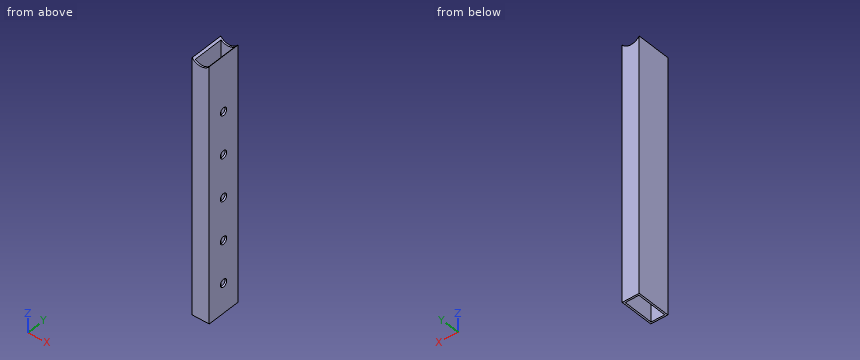
```python
from build123d import *

# Parameters (mm, degrees)
SKETCH_1_W          = 20
SKETCH_1_H          = 40
SKETCH_1_W_2        = 16
SKETCH_1_H_2        = 36
EXTRUDE_1_DEPTH     = 300
SKETCH_2_R          = 12.5
CUT_EXTRUDE_1_DEPTH = 40
SKETCH_3_R          = 4.5
CUT_EXTRUDE_2_DEPTH = 2


with BuildPart() as part:
    # Эскиз1 → Бобышка-Вытянуть1 (new body)
    with BuildSketch(Plane.XY):
        Rectangle(SKETCH_1_W, SKETCH_1_H)
        Rectangle(SKETCH_1_W_2, SKETCH_1_H_2, mode=Mode.SUBTRACT)
    extrude(amount=EXTRUDE_1_DEPTH)

    # Эскиз2 → Вырез-Вытянуть1 (cut)
    with BuildSketch(Plane(origin=(0, 20, 0), x_dir=(1, 0, 0), z_dir=(0, 1, 0))):
        with Locations((0, -307.5)):
            Circle(SKETCH_2_R)
    extrude(amount=-CUT_EXTRUDE_1_DEPTH, mode=Mode.SUBTRACT)

    # Эскиз3 → Вырез-Вытянуть2 (cut)
    with BuildSketch(Plane(origin=(10, 0, 0), x_dir=(0, 0, -1), z_dir=(1, 0, 0))):
        with Locations(Location((-35, 0, 0), (0, 0, 90))):  # turned: the seam where the file's is
            Circle(SKETCH_3_R)
        with Locations(Location((-85, 0, 0), (0, 0, 90))):  # turned: the seam where the file's is
            Circle(SKETCH_3_R)
        with Locations(Location((-135, 0, 0), (0, 0, 90))):  # turned: the seam where the file's is
            Circle(SKETCH_3_R)
        with Locations(Location((-185, 0, 0), (0, 0, 90))):  # turned: the seam where the file's is
            Circle(SKETCH_3_R)
        with Locations(Location((-235, 0, 0), (0, 0, 90))):  # turned: the seam where the file's is
            Circle(SKETCH_3_R)
    extrude(amount=-CUT_EXTRUDE_2_DEPTH, mode=Mode.SUBTRACT)


solid = part.part
```
Part model, mm, in its own coordinate system. Give positions to 0.01 mm unless a question says otherwise; leave off trailing zeros. Write each loop counter-clockwise with the first axis right and the second up, starting at its lowest first coordinate (ties: lowest second). Pieces come first, ordered by that corner, then holes. Notation, with made-up numbers: (18, 8) -> (74, 8) arc R27 cw to (74, 35) -> close; hole circle Ø10 at (28.5, 87). An arc over 180 degrees is marked (long way). Put each result on its own line as item: value. Start each with the question number.
Item 1: Cut at C-C (z = 275.5). List the corners of the cut face in (x, y).
Item 2: Cut at A-A (y = 0). List the corners of the cut face in (x, z).
Item 3: Cut at B-B (x = -0.5). List the corners of the cut face in (y, z).
Item 4: Cut at D-D (z = 35). List the corners of the cut face in (x, y), then the cut area to 3 significant figures.
Item 5: Wall check: L1, parallel to Z at x = 9.4, y = 0; L2, parallel to X at y = -15, z = 70.5; L3, parallel to Y at x = -1.5, z = 201.5. Give the ranges that are in metal, low to high. Write a range as [from, to].
Answer list:
1. outline: (-10, -20) -> (10, -20) -> (10, 20) -> (-10, 20) -> close; hole (-8, -18) -> (8, -18) -> (8, 18) -> (-8, 18) -> close
2. outline: (-10, 0) -> (-8, 0) -> (-8, 297.9) arc R12.5 cw to (-10, 300) -> close; (8, 0) -> (10, 0) -> (10, 30.5) -> (8, 30.5) -> close; (8, 39.5) -> (10, 39.5) -> (10, 80.5) -> (8, 80.5) -> close; (8, 89.5) -> (10, 89.5) -> (10, 130.5) -> (8, 130.5) -> close; (8, 139.5) -> (10, 139.5) -> (10, 180.5) -> (8, 180.5) -> close; (8, 189.5) -> (10, 189.5) -> (10, 230.5) -> (8, 230.5) -> close; (8, 239.5) -> (10, 239.5) -> (10, 300) arc R12.5 cw to (8, 297.9) -> close
3. outline: (-20, 0) -> (-18, 0) -> (-18, 295.01) -> (-20, 295.01) -> close; (18, 0) -> (20, 0) -> (20, 295.01) -> (18, 295.01) -> close
4. outline: (-10, -20) -> (10, -20) -> (10, -4.5) -> (8, -4.5) -> (8, -18) -> (-8, -18) -> (-8, 18) -> (8, 18) -> (8, 4.5) -> (10, 4.5) -> (10, 20) -> (-10, 20) -> close
4. area: 206 mm2
5. L1: z = [0, 30.5], [39.5, 80.5], [89.5, 130.5], [139.5, 180.5], [189.5, 230.5], [239.5, 299.26]
5. L2: x = [-10, -8], [8, 10]
5. L3: y = [-20, -18], [18, 20]
